Source: CAD feature listing. Evaluate the final solid. Frame: model axes, mm. A direction names the side the tool comes from. Coordinates: 2 decimals unless noted, no trailing zeros. Write each loop counter-clockwise with the first axis right and the second up, starting at its lowest first coordinate (ties: lowest second). Pieces come first, ordered by that corner, then holes. Notation, with made-up numbers: (-20.5, 76) -> (-13.5, 76) arc R23 cw to (-13.5, 107) -> close; hole circle Ø10 at (74, -12). An arc over 180 degrees is marked (long way). One line per item, written item: value. Start each with the question number.
1. Mould query, pull axis Y, two halves, no side actions, for faces 5 (the flat face through (8, 1, -55)), 6 (the cylindrical face through (-8.67, -39.05, -52.49)), 7 (the cylindrical face through (26.52, 17.44, 52.54)), 8 (the cylindrical face through (1.34, 32.11, 52.54)). Classes: released by +Y, released by -Y, zero draft, split by the parting line, or undercut.
2. First-contact query: P1, Ø1.5, axis at x = -19, z = -6, coming from the -Y side; P2, Ø6.5, axis at x = 0, y = -30, coming from the -Z side; P3, Ø10, axis at y = 9, z = -18, coming from the +X side; P4, Ø8, axis at x = -16, z = 29.5, coming from the -Y side. Flat tips, straight axial feed; report the tip coordinate or a pass-through.
3. Access query for faces 1 (the cylindrical face through (-4.336, -19.524, 0.7)), 2 (the cylindrical face through (28.29, -15.96, 52.54)), 3 (the flat face through (1, 3, -51.419)), 4 (the flat face through (1, 3, 51.419)). Directions: +Z, -Z, +X, -X, +Y, -Y. A direction counts if a zero-diameter tool reaches every point of the face in a straight line with its end or side. Return the directions, or none.
4. Line query: line 1 (Y direction, x = 0, z = -52); line 2 (Z direction, x = -28.5, y = 14); line 3 (Y direction, x = 0, z = -51). Output: solid intervals per line, ascending.
5. Section query A-A, the plane x = 0. State how many separate pieces and enclosed holes the cut face has, and give its area (3 significant figures).
6. Section query B-B, the plane z = -33. Output: boundary loops of the cut face in (x, y).
from build123d import *

# Parameters (mm, degrees)
SKETCH1_R                = 20
BOSS_EXTRUDE1_DEPTH      = 50
SKETCH3_R                = 40
BOSS_EXTRUDE2_DEPTH      = 5
CHAMFER1_SIZE            = 2
SKETCH5_R                = 2.5
CUT_EXTRUDE1_DEPTH       = 120.268604419
CIRPATTERN1_COUNT        = 6
FILLET2_R                = 3
MIRROR3_COPY_1_SKETCH_R  = 2.5
MIRROR3_COPY_1_DEPTH     = 120.268604419
MIRROR3_COPY_2_SKETCH_R  = 2.5
MIRROR3_COPY_2_DEPTH     = 120.268604419
MIRROR3_COPY_3_SKETCH_R  = 2.5
MIRROR3_COPY_3_DEPTH     = 120.268604419
MIRROR3_COPY_4_SKETCH_R  = 2.5
MIRROR3_COPY_4_DEPTH     = 120.268604419
MIRROR3_COPY_5_SKETCH_R  = 2.5
MIRROR3_COPY_5_DEPTH     = 120.268604419
CHAMFER1_OF_MIRROR3_SIZE = 2
FILLET2_OF_MIRROR3_R     = 3


with BuildPart() as part:
    # Sketch1 → Boss-Extrude1 (new, symmetric)
    with BuildSketch(Plane.XY):
        Circle(SKETCH1_R)
    boss_extrude1 = extrude(amount=BOSS_EXTRUDE1_DEPTH, both=True)

    # Sketch3 → Boss-Extrude2 (add)
    with BuildSketch(Plane.XY.offset(50)):
        Circle(SKETCH3_R)
    boss_extrude2 = extrude(amount=BOSS_EXTRUDE2_DEPTH)

    # Chamfer1
    chamfer1_edges = [part.edges().sort_by_distance(p)[0] for p in [
        (-40, 0, 50),
        (-40, 0, 55),
    ]]
    chamfer(chamfer1_edges, length=CHAMFER1_SIZE)

    # Sketch5 → Cut-Extrude1 (cut, through all)
    with BuildSketch(Plane.XY.offset(55)):
        with Locations((0, 30)):
            Circle(SKETCH5_R)
    cut_extrude1 = extrude(amount=-CUT_EXTRUDE1_DEPTH, mode=Mode.SUBTRACT)

    # CirPattern1: Cut-Extrude1 ×6 about axis
    cirpattern1_axis = Axis((0, 0, 0), (0, 0, 1))
    for i in range(1, CIRPATTERN1_COUNT):
        add(cut_extrude1.rotate(cirpattern1_axis, i * 360 / CIRPATTERN1_COUNT), mode=Mode.SUBTRACT)

    # Fillet2
    fillet2_edges = [part.edges().sort_by_distance(p)[0] for p in [
        (-38, 0, 50),
    ]]
    fillet(fillet2_edges, radius=FILLET2_R)

    # Sketch8 → CBORE for #12 Binding Head Machine Screw1 (revolve, cut)
    with BuildSketch(Plane(origin=(0, 0, 55), x_dir=(0, -1, 0), z_dir=(1, 0, 0))):
        Polygon((0, 0), (0, 110), (2.8067, 110), (2.8067, 3.5814), (5.95376, 3.5814), (5.95376, 0.635), (6.58876, 0), align=None)
    cbore_for_12_binding_head_machine_screw = revolve(axis=Axis((0, 0, 61.35), (0, 0, -1)), mode=Mode.SUBTRACT)

    # Mirror3: Boss-Extrude1, Boss-Extrude2, Cut-Extrude1, CBORE for #12 Binding Head Machine Screw1 across plane
    add(boss_extrude1.mirror(Plane.XY))
    add(boss_extrude2.mirror(Plane.XY))
    add(cut_extrude1.mirror(Plane.XY), mode=Mode.SUBTRACT)
    add(cbore_for_12_binding_head_machine_screw.mirror(Plane.XY), mode=Mode.SUBTRACT)

    # Mirror3 copy 1 sketch → Mirror3 copy 1 (cut, through all)
    with BuildSketch(Plane(origin=(0, 0, -55), x_dir=(0.5000000000000001, 0.8660254037844386, 0), z_dir=(0, 0, -1))):
        with Locations((0, -30)):
            Circle(MIRROR3_COPY_1_SKETCH_R)
    extrude(amount=-MIRROR3_COPY_1_DEPTH, mode=Mode.SUBTRACT)

    # Mirror3 copy 2 sketch → Mirror3 copy 2 (cut, through all)
    with BuildSketch(Plane(origin=(0, 0, -55), x_dir=(-0.4999999999999998, 0.8660254037844387, 0), z_dir=(0, 0, -1))):
        with Locations((0, -30)):
            Circle(MIRROR3_COPY_2_SKETCH_R)
    extrude(amount=-MIRROR3_COPY_2_DEPTH, mode=Mode.SUBTRACT)

    # Mirror3 copy 3 sketch → Mirror3 copy 3 (cut, through all)
    with BuildSketch(Plane(origin=(0, 0, -55), x_dir=(-1, 0, 0), z_dir=(0, 0, -1))):
        with Locations((0, -30)):
            Circle(MIRROR3_COPY_3_SKETCH_R)
    extrude(amount=-MIRROR3_COPY_3_DEPTH, mode=Mode.SUBTRACT)

    # Mirror3 copy 4 sketch → Mirror3 copy 4 (cut, through all)
    with BuildSketch(Plane(origin=(0, 0, -55), x_dir=(-0.5000000000000004, -0.8660254037844384, 0), z_dir=(0, 0, -1))):
        with Locations((0, -30)):
            Circle(MIRROR3_COPY_4_SKETCH_R)
    extrude(amount=-MIRROR3_COPY_4_DEPTH, mode=Mode.SUBTRACT)

    # Mirror3 copy 5 sketch → Mirror3 copy 5 (cut, through all)
    with BuildSketch(Plane(origin=(0, 0, -55), x_dir=(0.5000000000000001, -0.8660254037844386, 0), z_dir=(0, 0, -1))):
        with Locations((0, -30)):
            Circle(MIRROR3_COPY_5_SKETCH_R)
    extrude(amount=-MIRROR3_COPY_5_DEPTH, mode=Mode.SUBTRACT)

    # Chamfer1 of Mirror3
    chamfer1_of_mirror3_edges = [part.edges().sort_by_distance(p)[0] for p in [
        (-40, 0, -50),
        (-40, 0, -55),
    ]]
    chamfer(chamfer1_of_mirror3_edges, length=CHAMFER1_OF_MIRROR3_SIZE)

    # Fillet2 of Mirror3
    fillet2_of_mirror3_edges = [part.edges().sort_by_distance(p)[0] for p in [
        (-38, 0, -50),
    ]]
    fillet(fillet2_of_mirror3_edges, radius=FILLET2_OF_MIRROR3_R)


solid = part.part
Computed values:
1. face 5: zero draft
1. face 6: split by the parting line
1. face 7: undercut
1. face 8: undercut
2. P1: stops at y = -8.18
2. P2: stops at z = -55
2. P3: stops at x = 19.6
2. P4: stops at y = -16
3. face 1: none
3. face 2: +Z, -Z
3. face 3: -Z
3. face 4: +Z
4. line 1: y = -40 to -32.5, -27.5 to -5.95, 5.95 to 27.5, 32.5 to 40
4. line 2: z = -55 to -50, 50 to 55
4. line 3: y = -39 to -32.5, -27.5 to -2.81, 2.81 to 27.5, 32.5 to 39
5. separate pieces: 6
5. enclosed holes: 0
5. area: 4,020 mm²
6. outline: circle Ø40 at (0, 0); hole circle Ø5.61 at (0, 0)
